The model under review builds one solid part; all positions refer to its coordinate system, in mm. Round coordinates to 2 decimals unless told otherwise and drop trailing zeros. Write each loop counter-clockwise with the first axis right and the second up, starting at its lowest first coordinate (ties: lowest second). Pieces come first, ordered by that corner, then holes. Notation, with made-up numbers: (70.5, 7) -> (114.5, 7) arc R17 cw to (114.5, 24) -> close; hole circle Ø5 at (-4.5, 59). An arc over 180 degrees is marked (long way). Return JSON: item names as keys, results as strings. Group by question number.
1. For line 1 along X through (y, z) = (-36, 2.9); line 2 along Y through (x, z) = (-27, 3.85); line 3 along X through (y, z) = (-37.5, 1.7), list the stretches that pass through material, from the lowest coordinate up. Write a range as from..to.
2. Take a section at B-B, the plane x = 38.5. Write out the cut boundary in (y, z).
3. Take a section at A-A, the plane y = 0. Write out the cut boundary in (x, z), then the cut area to 3 significant figures.
4. Take a section at D-D, the plane y = -30. Write out the cut boundary in (x, z).
5. Take a section at C-C, the plane z = 1.35. Give the number of separate pieces and of enclosed holes in the cut face, then the cut area to 3 significant figures.
6. Clearance check with flat-ended pins moving along their axes: P1, Ø4.5, axis at x = 39.38, y = 10.55, coming from the +Z side; P2, Ø2, axis at y = 11.5, z = 2.5, coming from the -X side. State where each tip first meets the part, or that it passes through.
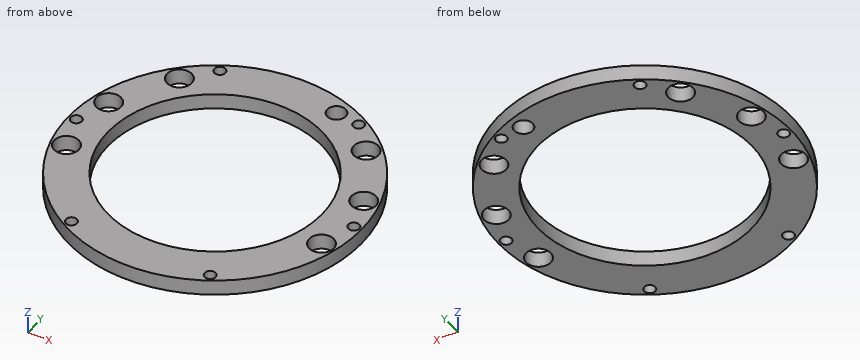
Autodesk Inventor part; units mm, degrees
ref_plane "YZ Plane" through (0, 0, 0) normal (1, 0, 0) x (0, 1, 0)
ref_plane "XZ Plane" through (0, 0, 0) normal (0, 1, 0) x (-1, 0, 0)
ref_plane "XY Plane" through (0, 0, 0) normal (0, 0, 1) x (1, 0, 0)
sketch "Sketch1" plane through (0, 0, 0) normal (0, 0, 1) x (1, 0, 0)
  circle A0 centre (0, 0) radius 45.212
  line L0 (0, 0) -> (21.4313, 37.12)
  line L1 (0, 0) -> (42.8625, 0) construction
  circle A1 centre (21.4313, 37.12) radius 1.7145
  circle A2 centre (-21.4312, 37.12) radius 1.7145
  circle A3 centre (-42.8625, 0) radius 1.7145
  circle A4 centre (-21.4313, -37.12) radius 1.7145
  circle A5 centre (21.4312, -37.12) radius 1.7145
  circle A6 centre (42.8625, 0) radius 1.7145
  dimension "d0" = 90.424
  dimension "d1" = 42.8625
  dimension "d2" = 60
  dimension "d3" = 3.429
  dimension "d6" = 360
extrude "Extrusion1" add sketch "Sketch1" along normal blind 4.7625
sketch "Sketch2" plane through (0, 0, 4.7625) normal (0, 0, 1) x (1, 0, 0)
  circle A0 centre (0, 0) radius 33.02
  dimension "d10" = 66.04
extrude "Extrusion2" cut sketch "Sketch2" against normal blind 25.4
sketch "Sketch8" plane through (0, 0, 4.7625) normal (0, 0, 1) x (1, 0, 0)
  circle A0 centre (0, 0) radius 33.02
  circle A1 centre (42.8625, 0) radius 1.7145
  circle A2 centre (21.4312, -37.12) radius 1.7145
  circle A3 centre (-21.4313, -37.12) radius 1.7145
  circle A4 centre (-42.8625, 0) radius 1.7145
  circle A5 centre (-21.4312, 37.12) radius 1.7145
  circle A6 centre (21.4313, 37.12) radius 1.7145
  circle A7 centre (0, 0) radius 45.212
  circle A8 centre (0, 0) radius 38.1
  circle A9 centre (39.3779, 10.5513) radius 3.81
  circle A10 centre (39.3779, 10.5513) radius 2.4447
  line L0 (0, 0) -> (39.3779, 10.5513)
  line L1 (0, 0) -> (36.2951, 20.955)
  line L2 (0, 0) -> (41.91, 0) construction
  circle A11 centre (36.2951, 20.955) radius 1.5875
  line L3 (0, 0) -> (0, 9.3613)
  circle A12 centre (39.3779, -10.5513) radius 3.81
  circle A13 centre (-39.3779, 10.5513) radius 3.81
  circle A14 centre (-39.3779, -10.5513) radius 3.81
  circle A15 centre (28.8266, 28.8266) radius 3.81
  line L4 (21.4313, 37.12) -> (0, 0)
  line L5 (0, 0) -> (28.8266, 28.8266)
  circle A16 centre (-28.8266, 28.8266) radius 3.81
  dimension "d37" = 76.2
  dimension "d38" = 7.62
  dimension "d39" = 4.8895
  dimension "d40" = 40.767
  dimension "d42" = 41.91
  dimension "d43" = 30
  dimension "d44" = 3.175
  dimension "d45" = 15
  dimension "d49" = 7.62
  dimension "d50" = 15
  dimension "d51" = 40.767
extrude "Extrusion6" cut sketch "Sketch8" against normal blind 25.4 contours L0 A8 A9 | A9 A8 L0 | A10 | A9 A8 | A12 A8 | A8 A12 | A13 A8 | A8 A13 | A14 A8 | A8 A14
extrude "Extrusion7" cut sketch "Sketch8" against normal blind 25.4 contours L5 A8 A15 | A15 A8 L5 | A15 A8 | A16 A8 | A8 A16
sketch "Sketch11" plane through (0, 0, 4.7625) normal (0, 0, 1) x (1, 0, 0)
  circle A0 centre (13.8997, 38.1891) radius 2.8575
  line L0 (0, 0) -> (13.8997, 38.1891) construction
  line L1 (0, 0) -> (40.64, 0) construction
  dimension "d55" = 5.715
  dimension "d56" = 70
  dimension "d57" = 40.64
extrude "Extrusion8" cut sketch "Sketch11" against normal through all
equation "\"d49\" = d38"
equation "\"d50\" = d45"
equation "\"d51\" = d40"
properties part number "forwardBallastSealingWallDisc" material "Aluminum 6061"
Output:
{
 "1": {"line 1": "x = -27.35..-22.73, -20.13..20.13, 22.73..27.35", "line 2": "y = -36.26..-19.01, 19.01..25.48, 32.17..36.26", "line 3": "x = -25.26..-23.1, -19.76..19.76, 23.1..25.26"},
 "2": {"outline": "(-23.7, 0) -> (-14.26, 0) -> (-14.26, 4.76) -> (-23.7, 4.76) -> close; (-6.84, 0) -> (6.84, 0) -> (6.84, 4.76) -> (-6.84, 4.76) -> close; (14.26, 0) -> (23.7, 0) -> (23.7, 4.76) -> (14.26, 4.76) -> close"},
 "3": {"outline": "(-45.21, 0) -> (-44.58, 0) -> (-44.58, 4.76) -> (-45.21, 4.76) -> close; (-41.15, 0) -> (-33.02, 0) -> (-33.02, 4.76) -> (-41.15, 4.76) -> close; (33.02, 0) -> (41.15, 0) -> (41.15, 4.76) -> (33.02, 4.76) -> close; (44.58, 0) -> (45.21, 0) -> (45.21, 4.76) -> (44.58, 4.76) -> close", "area": "83.5 mm^2"},
 "4": {"outline": "(-33.82, 0) -> (-13.8, 0) -> (-13.8, 4.76) -> (-33.82, 4.76) -> close; (13.8, 0) -> (33.82, 0) -> (33.82, 4.76) -> (13.8, 4.76) -> close"},
 "5": {"separate pieces": "1", "enclosed holes": "14", "area": "2,640 mm^2"},
 "6": {"P1": "passes through", "P2": "stops at x = -43.98"}
}
